```python
from build123d import *

# Parameters (mm, degrees)
CYLINDER004_R     = 1.25
CYLINDER004_DEPTH = 10
CYLINDER005_R     = 1.25
CYLINDER005_DEPTH = 10
CYLINDER013_R     = 1
CYLINDER013_DEPTH = 4.2
CYLINDER002_R     = 2.37
CYLINDER002_DEPTH = 2.36
BOX003_W          = 10.2
BOX003_H          = 28
BOX003_DEPTH      = 4.2
CYLINDER006_R     = 6.65
CYLINDER006_DEPTH = 4.2
BOX005_W          = 16.200001
BOX005_H          = 10
BOX005_DEPTH      = 4.2


with BuildPart() as cylinder004:
    # Cylinder004 → Cylinder004 (new body)
    with BuildSketch(Plane(origin=(5, 32, -3), x_dir=(1, 0, 0), z_dir=(0, 0, 1))):
        Circle(CYLINDER004_R)
    extrude(amount=CYLINDER004_DEPTH)


with BuildPart() as cylinder005:
    # Cylinder005 → Cylinder005 (new body)
    with BuildSketch(Plane(origin=(-5, 32, -3), x_dir=(1, 0, 0), z_dir=(0, 0, 1))):
        Circle(CYLINDER005_R)
    extrude(amount=CYLINDER005_DEPTH)


with BuildPart() as cylinder013:
    # Cylinder013 → Cylinder013 (new body)
    with BuildSketch(Plane.XY):
        Circle(CYLINDER013_R)
    extrude(amount=CYLINDER013_DEPTH)


with BuildPart() as fusion005002:
    # Cylinder002 → Cylinder002 (new body)
    with BuildSketch(Plane.XY):
        Circle(CYLINDER002_R)
    extrude(amount=CYLINDER002_DEPTH)

    # Fusion005002: union Cylinder004, Cylinder005, Cylinder013
    add(cylinder004.part)
    add(cylinder005.part)
    add(cylinder013.part)


with BuildPart() as box003:
    # Box003 → Box003 (new body)
    with BuildSketch(Plane(origin=(-5, 4, 0), x_dir=(1, 0, 0), z_dir=(0, 0, 1))):
        with Locations((5.1, 14)):
            Rectangle(BOX003_W, BOX003_H)
    extrude(amount=BOX003_DEPTH)


with BuildPart() as cylinder006:
    # Cylinder006 → Cylinder006 (new body)
    with BuildSketch(Plane.XY):
        Circle(CYLINDER006_R)
    extrude(amount=CYLINDER006_DEPTH)


with BuildPart() as horn:
    # Box005 → Box005 (new body)
    with BuildSketch(Plane(origin=(-8.1, 27, 0), x_dir=(1, 0, 0), z_dir=(0, 0, 1))):
        with Locations((8.100001, 5)):
            Rectangle(BOX005_W, BOX005_H)
    extrude(amount=BOX005_DEPTH)

    # Fusion003: union Box003, Cylinder006
    add(box003.part)
    add(cylinder006.part)

    # Cut002002003: cut Fusion005002
    add(fusion005002.part, mode=Mode.SUBTRACT)


solid = horn.part
```
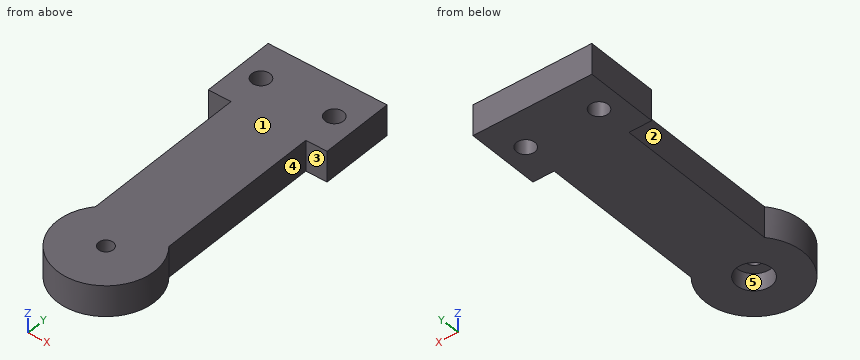
Build history of the part. All positions in model axes, mm. Face numbers are marked on the shaded views. A direction names the side the tool comes from. Give positions to 0.01 mm unless a question says otherwise; leave off trailing zeros. Order: outer loops, then holes, each group sorted by start corner. A loop starts at its lowest first (then second) coordinate and runs counter-clockwise, first axis right, second up. Notation, with made-up numbers: M -20.5,-2.5 L -7.5,-2.5 A5 ccw -7.5,4.5 Z; hole C 15,42.25 d3. An arc over 180 degrees is marked long. Return JSON: item names as keys, results as strings.
Q1. Band-saw the part on A-A (y = 0). Give the cut face in (x, z).
Answer list:
{"outline": "M -6.65,0 L -2.37,0 L -2.37,2.36 L -1,2.36 L -1,4.2 L -6.65,4.2 Z; M 1,2.36 L 2.37,2.36 L 2.37,0 L 6.65,0 L 6.65,4.2 L 1,4.2 Z"}
Q2. Wall check: probe 1 along X at (y, z) = (32, 2.6); probe 2 along Y at (x, z) = (0, 3.15); probe 3 along X at (y, z) = (0, 3.65). Give the ranges that are in metal, low to high. Write a range as from..to.
Answer list:
{"probe 1": "x = -8.1..-6.25, -3.75..3.75, 6.25..8.1", "probe 2": "y = -6.65..-1, 1..37", "probe 3": "x = -6.65..-1, 1..6.65"}
Q3. Band-saw the part on C-C (z = 1.05). Give the cut face in (x, y).
Answer list:
{"outline": "M -8.1,27 L -5,27 L -5,4.38 A6.65 ccw long 5.2,4.15 L 5.2,27 L 8.1,27 L 8.1,37 L -8.1,37 Z; hole C -5,32 d2.5; hole C 0,0 d4.74; hole C 5,32 d2.5"}
Q4. Band-saw the part on D-D (y = 21). Give the cut face in (x, z), then the cut area to 3 significant figures.
Answer list:
{"outline": "M -5,0 L 5.2,0 L 5.2,4.2 L -5,4.2 Z", "area": "42.8 mm^2"}
Q5. Two-plate mould, pull along X, no slides. Class the marked faces 3, 4 and 5: pulls with the +X half, pulls with the -X half, needs draft (parallel to the pull), parting line crosses it, or undercut.
Answer list:
{"face 3": "needs draft", "face 4": "pulls with the +X half", "face 5": "undercut"}
Q6. Band-saw the part on B-B (x = 0). Give the cut face in (y, z).
Answer list:
{"outline": "M -6.65,0 L -2.37,0 L -2.37,2.36 L -1,2.36 L -1,4.2 L -6.65,4.2 Z; M 1,2.36 L 2.37,2.36 L 2.37,0 L 37,0 L 37,4.2 L 1,4.2 Z"}
Q7. 3-axis set-ups, long thin cutter, end or side, ignore diameter. For the marked faces 1 and 2: which of +Z, -Z, +X, -X, +Y, -Y reach the whole face in a straight line?
Answer list:
{"face 1": "+Z, +X, -X, +Y, -Y", "face 2": "+Z, -Z, -X"}
Q8. Flat gauge pins, fed straight in: pin 1 (1 mm diameter, centred on x = -4, z = 1.5, fed in from -Y); pin 2 (2.5 mm diameter, centred on x = 0, y = 0, fed in from -Z); pin 3 (2.5 mm diameter, centred on x = 6.5, z = 1.5, fed in from -Y). Where does each tip first touch, or does it go through?
Answer list:
{"pin 1": "stops at y = -5.65", "pin 2": "stops at z = 2.36", "pin 3": "stops at y = -4.08"}
